from build123d import *
from build123d.topology import SkipClean

# Parameters (mm, degrees)
BASE_FLANGE1_DEPTH  = 38.1
CUT_EXTRUDE1_DEPTH  = 7.62
SKETCH9_R           = 3.3
BOSS_EXTRUDE1_DEPTH = 3.175
BOSS_EXTRUDE2_DEPTH = 7.62


# Sheet-metal steps are written as plain solids
with BuildPart() as part:
    # Sketch1 → Base-Flange1 (new body)
    with BuildSketch(Plane(origin=(0, 0, 0), x_dir=(1, 0, 0), z_dir=(0, 1, 0))):
        with BuildLine():
            Line((-657.047015903, -180.398251424), (-495.540915967, -159.83264605))
            ThreePointArc((-495.540915967, -159.83264605), (-466.529161595, -137.56639807), (-471.621526187, -101.351269827))
            Line((-471.621526187, -101.351269827), (-496.558145126, -69.722999952))
            Line((-496.558145126, -69.722999952), (-494.363477067, -68.198999952))
            Line((-494.363477067, -68.198999952), (-469.527179345, -99.700027778))
            ThreePointArc((-469.527179345, -99.700027778), (-464.060656724, -138.576037958), (-495.204030033, -162.478283377))
            Line((-495.204030033, -162.478283377), (-656.710129969, -183.043888751))
            ThreePointArc((-656.710129969, -183.043888751), (-764.987734735, -111.822063922), (-711.2, 6.090902363))
            Line((-711.2, 6.090902363), (-710.077660148, 3.671554877))
            ThreePointArc((-710.077660148, 3.671554877), (-762.424972114, -111.083730158), (-657.047015903, -180.398251424))
        make_face()
    extrude(amount=-BASE_FLANGE1_DEPTH)

    # Sketch7 → Cut-Extrude1 (cut)
    with BuildSketch(Plane(origin=(-711.2, 0, -6.090902363), x_dir=(1, 0, 0), z_dir=(0, 1, 0))):
        with BuildLine():
            Line((1.122339852, -2.419347486), (0, 0))
            ThreePointArc((0, 0), (-28.443609249, -19.854342865), (-48.352212426, -48.26))
            Line((-48.352212426, -48.26), (-45.400744677, -48.26))
            ThreePointArc((-45.400744677, -48.26), (-26.116771828, -21.302890058), (1.122339852, -2.419347486))
        make_face()
    extrude(amount=-CUT_EXTRUDE1_DEPTH, mode=Mode.SUBTRACT)

    # Sketch9 → Boss-Extrude1 (add)
    with BuildSketch(Plane(origin=(0, -11.93175668, 0), x_dir=(1, 0, 0), z_dir=(0, 1, 0))):
        with BuildLine():
            ThreePointArc((-751.074016673, -2.593523568), (-764.50540437, -3.617766971), (-763.481160967, -17.049154667))
            Line((-763.481160967, -17.049154667), (-751.193944793, -27.595167013))
            ThreePointArc((-751.193944793, -27.595167013), (-745.401952839, -20.024035331), (-738.912633033, -13.041347154))
            Line((-738.912633033, -13.041347154), (-751.074016673, -2.593523568))
        make_face()
        with Locations(Location((-757.27758882, -9.821339117, 0), (0, 0, 270))):
            Circle(SKETCH9_R, mode=Mode.SUBTRACT)
    extrude(amount=-BOSS_EXTRUDE1_DEPTH)

    # Sketch10 → Boss-Extrude2 (add)
    with SkipClean():  # the faces are left unmerged after this step: merging them gives an invalid solid
        with BuildSketch(Plane.XZ.offset(38.1)):
            with BuildLine():
                Line((-710.077660148, -3.671554877), (-711.2, -6.090902363))
                ThreePointArc((-711.2, -6.090902363), (-764.987734735, 111.822063922), (-656.710129969, 183.043888751))
                Line((-656.710129969, 183.043888751), (-575.957080001, 172.761086064))
                Line((-575.957080001, 172.761086064), (-576.293965935, 170.115448737))
                Line((-576.293965935, 170.115448737), (-657.047015903, 180.398251424))
                ThreePointArc((-657.047015903, 180.398251424), (-762.424972114, 111.083730158), (-710.077660148, -3.671554877))
            make_face()
        extrude(amount=BOSS_EXTRUDE2_DEPTH)


solid = part.part
Model file for the job. Use its own axes, mm. A direction names the side the tool comes from. Give positions to 0.01 mm unless a question says otherwise; leave off trailing zeros. Order: outer loops, then holes, each group sorted by start corner. A loop starts at its lowest first (then second) coordinate and runs counter-clockwise, first axis right, second up. Notation, with made-up numbers: (39, 15) - (96, 15) arc R27 ccw to (96, 34) - close; hole circle Ø6 at (34.5, 72.25). An arc over 180 degrees is marked (long way). Write item = value, one per line. Start each with the question number.
1. Cut at C-C, the plane x = -748. List the corners of the cut face in (y, z).
2. Cut at A-A, the plane y = -23.5. List the corners of the cut face in (x, z) (3 decimals), and give its area (3 significant figures).
3. Which spindle directions (+Z, -Z, +X, -X, +Y, -Y) get a long thin tool onto all of the face, cutting with end or side? Do faces 1 (the flat face through (-753, -15.107, 14)), 2 (the cylindrical face through (-761.874, -22.54, 112.926)), 3 (the flat face through (-489, -38.1, 159)). Say none if no direction does.
4. Probe line 1 along X through (y, z) = (-8, 98); line 2 along Z through (x, y) = (-732, -35.5); line 3 along X through (y, z) = (-18, 134). List the from-to ranges inside material, lowest first.
5. Drop flat-ended pins along their axis: P1, Ø8, axis at x = -627, y = -29, coming from the +Z side; P2, Ø2, axis at x = -509, y = -9.5, coming from the -Z side; P3, Ø4, axis at x = -647, y = -24.5, coming from the -Z side; P4, Ø13.5, axis at x = -748.5, z = 17.5, coming from the -Y side. Give the stop position or say it passes through.
6. Cut at D-D, the plane z = 85. List the corners of the cut face in (x, y), and give its area (3 significant figures).
7. Cut at B-B, the plane z = 114.5. List the corners of the cut face in (x, y).
8. Two-plate mould, pull along Z, no slides. Class faces 4 (the flat face through (-482.12, -18.78, 83.73)), 5 (the flat face through (-757.42, -13.5, 22.25)), 6 (the cylindrical face through (-463.847, -18.783, 138.041)): pulls with the +Z half, pulls with the -Z half, needs draft (parallel to the pull), parting line crosses it, or undercut.
Taken from the geometry:
q1.outline = (-45.72, 23.24) - (-15.11, 23.24) - (-15.11, 5.23) - (-11.93, 5.23) - (-11.93, 23.24) - (-7.62, 23.24) - (-7.62, 27.69) - (-45.72, 27.69) - close; (-45.72, 140.81) - (0, 140.81) - (0, 145.27) - (-45.72, 145.27) - close
q2.outline = (-711.2, -6.091) - (-710.078, -3.672) arc R96.923 cw to (-657.047, 180.398) - (-495.541, 159.833) arc R36.298 cw to (-471.622, 101.351) - (-496.558, 69.723) - (-494.363, 68.199) - (-469.527, 99.7) arc R38.965 ccw to (-495.204, 162.478) - (-656.71, 183.044) arc R99.59 ccw to start
q2.area = 1,500 mm²
q3.face_1 = -Z, -X, -Y
q3.face_2 = +Y, -Y
q3.face_3 = +Z, -Z, +X, -Y
q4.line_1 = -767.93 to -765.23, -474.26 to -470.87
q4.line_2 = 6.88 to 10.35, 158.15 to 161.62
q4.line_3 = -755.56 to -752.47, -465.28 to -462.51
q5.P1 = 179.77
q5.P2 = 161.42
q5.P3 = 178.86
q5.P4 = -45.72
q6.outline = (-768.88, -45.72) - (-766.21, -45.72) - (-766.21, 0) - (-768.88, 0) - close; (-484.51, -38.1) - (-481.12, -38.1) - (-481.12, 0) - (-484.51, 0) - close
q6.area = 251 mm²
q7.outline = (-764.18, -45.72) - (-761.37, -45.72) - (-761.37, 0) - (-764.18, 0) - close; (-465.05, -38.1) - (-462.29, -38.1) - (-462.29, 0) - (-465.05, 0) - close
q8.face_4 = pulls with the -Z half
q8.face_5 = undercut
q8.face_6 = parting line crosses it
